Can you work these out from the model? Positions are in its coordinate system, mm. A direction names the side the tool comes from. Coordinates: 2 decimals unless noted, no trailing zeros. Write each loop counter-clockwise with the first axis right and the second up, starting at its lowest first coordinate (ties: lowest second). Pieces come first, ordered by that corner, then holes. Notation, with made-up numbers: M 45.25,-8 L 87.25,-8 A7 ccw 87.25,0 Z; hole C 7.5,85 d9. An arc over 180 degrees is marked long. Use one line per item in the form item = value. Start each with the question number.
```python
from build123d import *

# Parameters (mm, degrees)
F0_R     = 19
F1_DEPTH = 920
F2_R     = 8
F3_DEPTH = 30


with BuildPart() as f1:
    # F0 (on Top) → F1 (new body)
    with BuildSketch(Plane.XY):
        Circle(F0_R)
    extrude(amount=F1_DEPTH)

    # F2 (on Front) → F3 (join, symmetric)
    with BuildSketch(Plane.XZ):
        with Locations((0, 15)):
            Circle(F2_R)
    extrude(amount=F3_DEPTH, both=True)


solid = f1.part
```
1) Suppose I cut it at B-B on x = 0. Please give me the cut outline in (y, z), and give its area (3 significant figures).
2) Will these pins go through, and if not, where does the flat tip stop? pin 1 Ø6 at (y, z) = (11, 308.5) entering from +X; pin 2 Ø1 at (x, z) = (-8, 750.5) entering from -Y; pin 3 Ø3 at (y, z) = (14.5, 575.5) entering from -X.
3) Please list where these lines run through material, in increasing order: line 1 (Y direction, x = 2, z = 217); line 2 (X direction, y = -4, z = 518.5); line 3 (Y direction, x = 2.5, z = 644).
4) Suppose I cut it at A-A on z = 15. Please give me the cut outline in (x, y).
5) Suppose I cut it at C-C on z = 731.5. Please give me the cut outline in (x, y), and give its area (3 significant figures).
6) Which directions (+Z, -Z, +X, -X, +Y, -Y) give clear straight access to the entire face, cutting with the end or side of a thin tool? Please do faces 1 (the face through (7.63, 23.53, 17.4)), 2 (the face through (0, 0, 0)), 3 (the face through (-1.73, -23.71, 7.19)).
Computed values:
q1.outline = M -30,7 L -19,7 L -19,0 L 19,0 L 19,7 L 30,7 L 30,23 L 19,23 L 19,920 L -19,920 L -19,23 L -30,23 Z
q1.area = 35,300 mm²
q2.pin_1 = 17.23
q2.pin_2 = -17.46
q2.pin_3 = -13.86
q3.line_1 = -18.89 to 18.89
q3.line_2 = -18.57 to 18.57
q3.line_3 = -18.83 to 18.83
q4.outline = M -8,-30 L 8,-30 L 8,-17.23 A19 ccw 8,17.23 L 8,30 L -8,30 L -8,17.23 A19 ccw -8,-17.23 Z
q5.outline = C 0,0 d38
q5.area = 1,130 mm²
q6.face_1 = +Y
q6.face_2 = -Z, +X, -X, +Y, -Y
q6.face_3 = -Y
